Solid Edge part; units mm, degrees
sketch "Sketch1" plane through (0, 0, 0) normal (0, 0, 1) x (1, 0, 0)
  line L0 (24, -45) -> (24, 45)
  line L1 (24, 45) -> (-24, 45)
  line L2 (-24, 45) -> (-24, -45)
  line L3 (-24, -45) -> (24, -45)
extrude "Protrusion1" add sketch "Sketch1" along normal blind 103
sketch "Sketch2" plane through (0, -45, 51.5) normal (0, -1, 0) x (1, 0, 0)
  line L0 (6, 5.5) -> (24, 5.5)
  line L1 (24, 5.5) -> (24, 29.5)
  line L2 (24, 29.5) -> (6, 29.5)
  line L3 (6, 29.5) -> (6, 5.5)
  line L4 (24, -6.5) -> (6, -6.5)
  line L5 (6, -6.5) -> (6, -51.5)
  line L6 (6, -51.5) -> (24, -51.5)
  line L7 (24, -51.5) -> (24, -6.5)
extrude "Cutout1" cut sketch "Sketch2" against normal up to next
sketch "Sketch3" plane through (0, 0, 103) normal (0, 0, 1) x (1, 0, 0)
  line L0 (-24, 5) -> (-6, 5)
  line L1 (-6, 5) -> (-6, 45)
  line L2 (-6, 45) -> (-24, 45)
  line L3 (-24, 45) -> (-24, 5)
extrude "Cutout2" cut sketch "Sketch3" against normal up to next
sketch "Sketch4" plane through (-24, -20, 51.5) normal (-1, 0, 0) x (0, -1, 0)
  line L0 (-20, 51.5) -> (25, 15.5)
extrude "Cutout3" cut sketch "Sketch4" against normal up to next material side at (-24, -22.5312, 85.039)
sketch "Sketch5" plane through (0, 0, 0) normal (0, 0, 1) x (1, 0, 0)
  line L0 (-4, -29.3826) -> (-4, -20.0122)
  line L1 (-4, -20.0122) -> (-16, -20.0122)
  line L2 (-16, -20.0122) -> (-16, -29.3826)
  line L3 (-16, -29.3826) -> (-4, -29.3826)
extrude "Cutout4" cut sketch "Sketch5" along normal up to next
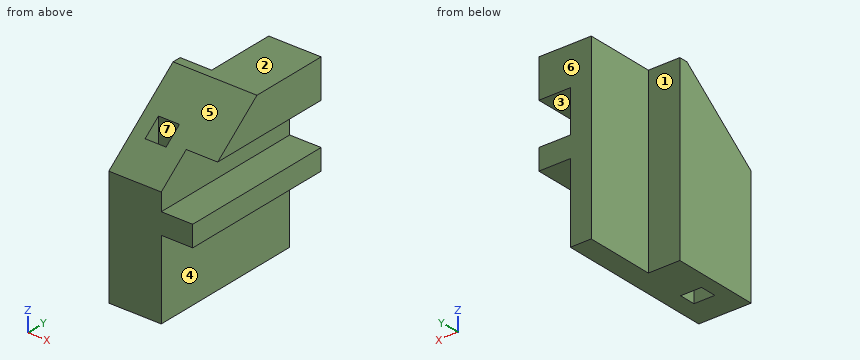
Geometry check sheet. Reference: the model listing, model coordinates, mm. Face numbers are marked on the shaded views. A direction names the side the tool comes from. Round coordinates to 2 decimals unless told otherwise and drop trailing zeros. Loops run counter-clockwise (first coordinate to the right, second up) from the corner with the lowest first, then second, coordinate; pieces in that order, holes last.
Item 1: Access from +Z, -Z, +X, -X, +Y, -Y to the whole of each face (thin tool, end or side, straight path). Record for the marked faces 1, 2, 3 and 4.
Item 2: Thickness scan on line 1 (Y direction, x = -8.5, z = 18); line 2 (X direction, y = -29, z = 71); line 3 (X direction, y = -14.5, z = 10). Record the ranges inside material, lowest first.
Item 3: Cross-section at B-B on z = 34. Record the boundary of the cut face in (x, y).
Item 4: Gauge pin test, flat ends, axial feed: pin 1 (3 mm diameter, centred on y = 10, z = 75, fed in from -X); pin 2 (5.5 mm diameter, centred on x = 18.5, y = -0.5, fed in from +Z); pin 3 (5.5 mm diameter, centred on x = 16.5, y = 8, fed in from -Z); pin 4 (10 mm diameter, centred on y = -0.5, z = 21.5, fed in from +X). Record the tip position at first contact, or that the pin passes through.
Item 5: Cross-section at C-C on y = 27. Record the boundary of the cut face in (x, z).
Item 6: Cross-section at A-A on x = 16.5. Record the boundary of the cut face in (y, z), then the cut area to 3 significant figures.
Item 7: Cross-section at D-D on x = -13.5. Record the boundary of the cut face in (y, z), then the cut area to 3 significant figures.
Item 8: Mould release check, pull along Y, two halves, no side actions. Record for the marked faces 5, 6 and 7: pulls with the +Y half, pulls with the -Y half, needs draft (parallel to the pull), parting line crosses it, or undercut.
Answer sheet:
1. face 1: +Z, -Z, -X, +Y
1. face 2: +Z, +X, -X, +Y, -Y
1. face 3: +X, +Y, -Y
1. face 4: -Z, +X, +Y, -Y
2. line 1: y = -45 to -29.38, -20.01 to 5
2. line 2: x = -24 to -16, -4 to 6
2. line 3: x = -24 to 6
3. outline: (-24, -45) - (6, -45) - (6, 45) - (-6, 45) - (-6, 5) - (-24, 5) - close; hole (-16, -29.38) - (-4, -29.38) - (-4, -20.01) - (-16, -20.01) - close
4. pin 1: stops at x = -6
4. pin 2: stops at z = 103
4. pin 3: stops at z = 45
4. pin 4: stops at x = 6
5. outline: (-6, 0) - (6, 0) - (6, 45) - (24, 45) - (24, 57) - (6, 57) - (6, 81) - (24, 81) - (24, 103) - (-6, 103) - close
6. outline: (-45, 45) - (45, 45) - (45, 57) - (-45, 57) - close; (-27.5, 81) - (45, 81) - (45, 103) - (0, 103) - close
6. area: 2,370 mm2
7. outline: (-45, 0) - (-29.38, 0) - (-29.38, 79.49) - (-45, 67) - close; (-20.01, 0) - (5, 0) - (5, 103) - (0, 103) - (-20.01, 86.99) - close
7. area: 3,560 mm2
8. face 5: pulls with the -Y half
8. face 6: pulls with the +Y half
8. face 7: undercut
